Could you check a few things on this drawing? It's one solid part, dimensions in mm from its lowest x, y, z. Coordinates: 2 decimals unless noted, no trailing zeros. Order: outer loops, then holes, each group sorted by start corner. A loop starts at its lowest first (then second) coordinate and runs counter-clockwise, first axis right, second up. Notation, with made-up numbers: (-15.75, 59.25) -> (28.25, 59.25) arc R7 cw to (28.25, 69.25) -> close; hole circle Ø5 at (64, 54). An arc over 180 degrees is marked (long way). Use a Markdown table: item, result. Add a question column.
1. Suppose I cut it at A-A, the plane y = 28.5. List the corners of the cut face in (x, z) for me.
2. For pin 1 Ø1 at (x, z) = (36.5, 0.5) entering from -Y, with a flat end and sliding along its axis, tell me the tip position at first contact or that it passes through.
3. If I drill on line 1 along Y through (x, z) = (28.5, 1.3); line 2 along Y through (x, z) = (11.5, 0.7) (1 decimal); line 3 along Y through (x, z) = (26.5, 1.35), over which ranges is the centre line in solid material (lowest first)? Write a range as from..to.
4. Suppose I cut it at D-D, the plane y = 41.5. List the corners of the cut face in (x, z) for me, then the cut area to 3 significant figures.
5. Suppose I cut it at C-C, the plane z = 1.2. State how many separate pieces and enclosed holes the cut face has, then the cut area to 3 significant figures.
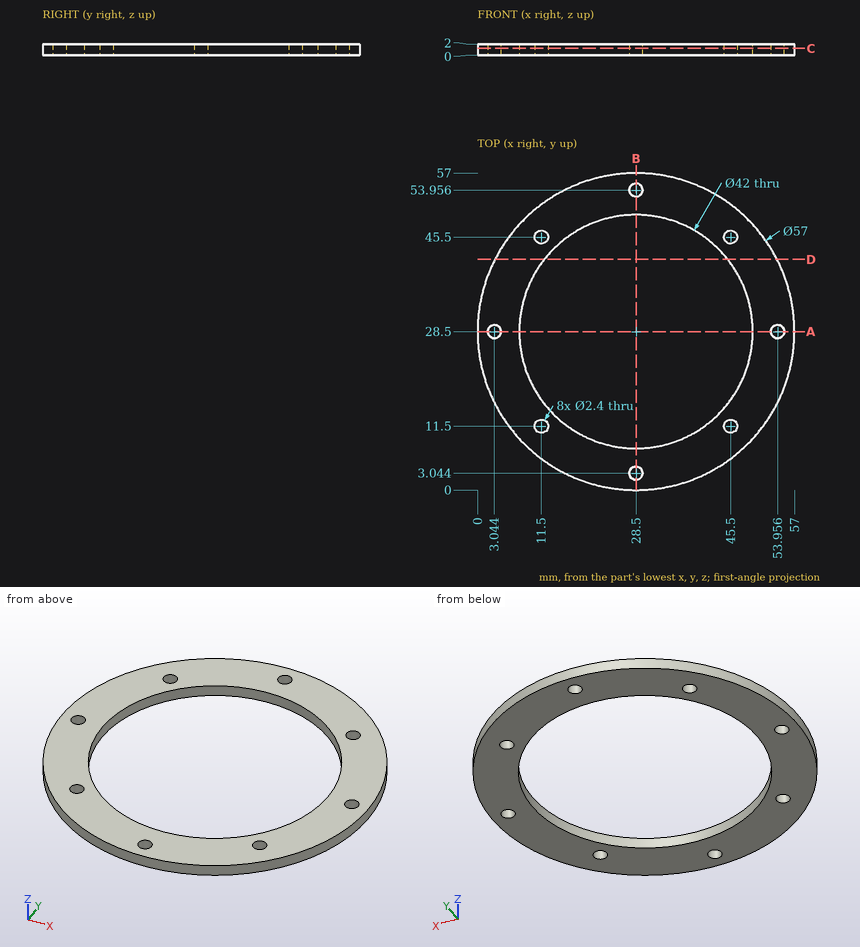
Worked out:
| question | item | result |
|---|---|---|
| 1 | outline | (0, 0) -> (1.84, 0) -> (1.84, 2) -> (0, 2) -> close; (4.24, 0) -> (7.5, 0) -> (7.5, 2) -> (4.24, 2) -> close; (49.5, 0) -> (52.76, 0) -> (52.76, 2) -> (49.5, 2) -> close; (55.16, 0) -> (57, 0) -> (57, 2) -> (55.16, 2) -> close |
| 2 | pin 1 | stops at y = 1 |
| 3 | line 1 | y = 0..1.84, 4.24..7.5, 49.5..52.76, 55.16..57 |
| 3 | line 2 | y = 5.6..10.3, 12.7..16.2, 40.8..44.3, 46.7..51.4 |
| 3 | line 3 | y = 0.07..7.6, 49.4..56.93 |
| 4 | outline | (3.14, 0) -> (12.01, 0) -> (12.01, 2) -> (3.14, 2) -> close; (44.99, 0) -> (53.86, 0) -> (53.86, 2) -> (44.99, 2) -> close |
| 4 | area | 35.5 mm² |
| 5 | separate pieces | 1 |
| 5 | enclosed holes | 9 |
| 5 | area | 1,130 mm² |
